Can you work these out from the model? Positions are in its coordinate system, mm. A direction names the side the tool comes from. Coordinates: 2 decimals unless noted, no trailing zeros. Order: outer loops, then holes, each group sorted by start corner. A loop starts at its lowest first (then second) coordinate and runs counter-clockwise, first axis right, second up. Notation, with made-up numbers: (49.25, 34) - (53.25, 34) arc R18 ccw to (53.25, 63) - close; hole circle Ø9 at (-31.75, 78.5). An arc over 180 degrees is marked (long way). Use a Markdown table: item, result. Add a question column.
(1) I want a section at D-D (z = 0.75). List the corners of the cut face in (x, y) for me.
(2) I want a section at C-C (z = -8.75). List the corners of the cut face in (x, y) for me.
(3) We'd pull the mould along Y, two halves only. Please class faces 1 (the cylindrical face through (-8.888, 28.338, -7.781)), 2 (the cylindrical face through (-19.6, -1.2, 2.1)), 3 (the flat face through (10, 11, -5)): pulls with the +Y half, pulls with the -Y half, needs draft (parallel to the pull), parting line crosses it, or undercut.
(4) I want a section at A-A (x = -18). List the corners of the cut face in (y, z) for me, and give its area (3 significant figures).
(5) I want a section at B-B (y = 0). List the corners of the cut face in (x, z) for me, and give its area (3 significant figures).
(6) If I drill on L1, parallel to Z at x = -0.5, y = -4; L2, parallel to Y at x = 0, z = 2.3; L3, parallel to Y at x = -1.5, z = 0.5, over which ranges is the centre line in solid material (lowest first)? Write a range as [from, to].
(7) On a 3-axis mill with a long thin cutter (end or side, diameter ignored), from which of +Z, -Z, +X, -X, +Y, -Y can I reach the whole of each face in a straight line? I mean faces 4 (the flat face through (-10, -10, 2)), 5 (the flat face through (1, 10, -10)), 6 (the flat face through (-20, 10, 2)). Say none if no direction works.
(8) For pin 1 Ø13 at (y, z) = (22, -10) entering from -X; pin 2 Ø10 at (x, y) = (-25.5, 9) entering from -Z; pin 3 Ø4.5 at (x, z) = (-22.5, 2.5) entering from +Y, each with a flat end and sliding along its axis, tell me the tip position at first contact or that it passes through.
```python
from build123d import *

# Parameters (mm, degrees)
SKETCH_1_W          = 40
SKETCH_1_H          = 20
SKETCH_1_R          = 2
EXTRUDE_1_DEPTH     = 4.1
SKETCH_2_W          = 20
SKETCH_2_H          = 20
EXTRUDE_2_DEPTH     = 24.1
SKETCH_3_R          = 2
CUT_EXTRUDE_1_DEPTH = 49.793544655


with BuildPart() as part:
    # 草图1 → 凸台-拉伸1 (new body)
    with BuildSketch(Plane.XY):
        with Locations((-10, 0)):
            Rectangle(SKETCH_1_W, SKETCH_1_H)
        Circle(SKETCH_1_R, mode=Mode.SUBTRACT)
    extrude(amount=EXTRUDE_1_DEPTH)

    # 草图2 → 凸台-拉伸2 (add)
    with BuildSketch(Plane.XY.offset(4.1)):
        with Locations((0, 20)):
            Rectangle(SKETCH_2_W, SKETCH_2_H)
    extrude(amount=-EXTRUDE_2_DEPTH)

    # 草图3 → 切除-拉伸1 (cut, through all)
    with BuildSketch(Plane.XY.offset(4.1)):
        with Locations((-18, 0)):
            Circle(SKETCH_3_R)
        with Locations((-30, 10)):
            Circle(SKETCH_3_R)
        with Locations((-3.589185504, 17.178371007)):
            Circle(SKETCH_3_R)
        with BuildLine():
            Line((-11.952534179, 30.433140022), (-10, 28))
            ThreePointArc((-10, 28), (-8.873826297, 28.347204553), (-8.138665231, 29.26826721))
            ThreePointArc((-8.138665231, 29.26826721), (0.312733547, 23.112455845), (10, 19.178371007))
            Line((10, 19.178371007), (10, 30))
            Line((10, 30), (-8, 30))
            ThreePointArc((-8, 30), (-9.78213348, 31.988098131), (-11.952534179, 30.433140022))
        make_face()
        with BuildLine():
            Line((-12, 10), (-10, 12))
            ThreePointArc((-10, 12), (-8.585786438, 8.585786438), (-12, 10))
        make_face()
    extrude(amount=-CUT_EXTRUDE_1_DEPTH, mode=Mode.SUBTRACT)


solid = part.part
```
Answers follow:
| question | item | result |
|---|---|---|
| 1 | outline | (-30, -10) - (10, -10) - (10, 19.18) arc R43 cw to (-8.14, 29.27) arc R2 cw to (-10, 28) - (-10, 12) arc R2 cw (long way) to (-12, 10) - (-28, 10) arc R2 cw to (-30, 8) - close; hole circle Ø4 at (-18, 0); hole circle Ø4 at (-3.59, 17.18); hole circle Ø4 at (0, 0) |
| 2 | outline | (-10, 12) arc R2 cw to (-8, 10) - (10, 10) - (10, 19.18) arc R43 cw to (-8.14, 29.27) arc R2 cw to (-10, 28) - close; hole circle Ø4 at (-3.59, 17.18) |
| 3 | face 1 | pulls with the +Y half |
| 3 | face 2 | undercut |
| 3 | face 3 | needs draft |
| 4 | outline | (-10, 0) - (-2, 0) - (-2, 4.1) - (-10, 4.1) - close; (2, 0) - (10, 0) - (10, 4.1) - (2, 4.1) - close |
| 4 | area | 65.6 mm² |
| 5 | outline | (-30, 0) - (-20, 0) - (-20, 4.1) - (-30, 4.1) - close; (-16, 0) - (-2, 0) - (-2, 4.1) - (-16, 4.1) - close; (2, 0) - (10, 0) - (10, 4.1) - (2, 4.1) - close |
| 5 | area | 131 mm² |
| 6 | L1 | z = [0, 4.1] |
| 6 | L2 | y = [-10, -2], [2, 23.29] |
| 6 | L3 | y = [-10, -1.32], [1.32, 24.18] |
| 7 | face 4 | +Z, -Z, +X, -X, -Y |
| 7 | face 5 | -Z, +X, -X, -Y |
| 7 | face 6 | +Z, -Z, -X, +Y |
| 8 | pin 1 | stops at x = -10 |
| 8 | pin 2 | stops at z = 0 |
| 8 | pin 3 | stops at y = 10 |
